Input: part model. Units: mm. Frame: model coordinates. Coordinates: 2 decimals unless noted, no trailing zeros. Loops run counter-clockwise (first coordinate to the right, second up) from the corner with the lowest first, then second, coordinate; pieces in that order, holes last. Notation, with made-up numbers: (-24, -2.5) -> (-7, -2.5) arc R16 ccw to (-7, 14.5) -> close; hole circle Ø7 at (-21.5, 49). An arc over 180 degrees is marked (long way). Put each result on its own line as item: value. Start each with the question number.
1) Cut plane C-C (x = -0.55). Return the cut outline in (y, z).
2) Material intervals for L1, parallel to Y at x = -0.9, z = -0.3; L2, parallel to Z at x = -1.5, y = -6; L3, parallel to Z at x = -1.95, y = 0.5, sorted ascending.
3) Contact query for flat-ended pins moving along their axis: P1, Ø1, axis at y = -3, z = 1.5, coming from the +X side; P2, Ø1, axis at x = 1.5, y = -12, coming from the +Z side; P3, Ø1.5, axis at y = -3.5, z = 0.5, coming from the -X side. Output: stop coordinate, or through.
4) Cut plane B-B (y = -17). Return the cut outline in (x, z), plus the area to 3 significant figures.
5) Cut plane A-A (z = 0). Return the cut outline in (x, y), plus the area to 3 significant figures.
6) Cut plane D-D (z = -1.7). Return the cut outline in (x, y), plus the area to 3 significant figures.
Autodesk Inventor part; units mm, degrees
ref_plane "YZ Plane" through (0, 0, 0) normal (1, 0, 0) x (0, 1, 0)
ref_plane "XZ Plane" through (0, 0, 0) normal (0, 1, 0) x (-1, 0, 0)
ref_plane "XY Plane" through (0, 0, 0) normal (0, 0, 1) x (1, 0, 0)
sketch "Sketch2" plane through (0, 0, 0) normal (0, 1, 0) x (-1, 0, 0)
  line L0 (0.8521, -2.0836) -> (-0.8521, -2.0836)
  line L1 (-0.8521, 2.0836) -> (0.8521, 2.0836)
  arc A0 (0.8521, -2.0836) -> (0.8521, 2.0836) centre (0, 0) ccw
  arc A1 (-0.8521, 2.0836) -> (-0.8521, -2.0836) centre (0, 0) ccw
  point P0 (0, -2.0836)
extrude "Extrusion1" add sketch "Sketch2" along normal blind 1.1906
sketch "Sketch3" plane through (0, 0, 0) normal (0, -1, 0) x (1, 0, 0)
  circle A0 centre (-1.6558, 0) radius 0.2977
  circle A1 centre (1.6558, 0) radius 0.2977
  arc A2 (0.8521, -2.0836) -> (0.8521, 2.0836) centre (0, 0) ccw
  arc A3 (-0.8521, 2.0836) -> (-0.8521, -2.0836) centre (0, 0) ccw
  point P0 (2.2511, 0)
  point P1 (-2.2511, 0)
  dimension "d6" = 0.5953
  dimension "d7" = 0.5953
  dimension "d8" = 0.5953
  dimension "d9" = 0.5953
extrude "Extrusion2" add sketch "Sketch3" along normal blind 33.5359
properties part number "PhotoResistor"
Results found:
1. outline: (0, -2.08) -> (1.19, -2.08) -> (1.19, 2.08) -> (0, 2.08) -> close
2. L1: y = 0 to 1.19
2. L2: z = -0.25 to 0.25
2. L3: z = -1.12 to 1.12
3. P1: passes through
3. P2: stops at z = 0.3
3. P3: stops at x = -1.95
4. outline: circle Ø0.6 at (-1.66, 0); circle Ø0.6 at (1.66, 0)
4. area: 0.557 mm2
5. outline: (-2.25, 0) -> (-1.95, 0) -> (-1.95, -33.54) -> (-1.36, -33.54) -> (-1.36, 0) -> (1.36, 0) -> (1.36, -33.54) -> (1.95, -33.54) -> (1.95, 0) -> (2.25, 0) -> (2.25, 1.19) -> (-2.25, 1.19) -> close
5. area: 45.3 mm2
6. outline: (-1.48, 0) -> (1.48, 0) -> (1.48, 1.19) -> (-1.48, 1.19) -> close
6. area: 3.51 mm2
